Input: part model. Units: mm. Frame: model coordinates. A direction names the side the tool comes from. Coordinates: 2 decimals unless noted, no trailing zeros. Order: outer loops, then holes, each group sorted by start corner. A loop starts at its lowest first (then second) coordinate and runs counter-clockwise, first axis right, second up. Notation, with made-up numbers: (54, 18) - (85, 18) arc R13 ccw to (85, 30) - close; hole circle Ø3 at (4, 7). An arc over 180 degrees is marked (long way). One line per question, with ' | ' between items.
from build123d import *

# Parameters (mm, degrees)
SKETCH1_W            = 91
SKETCH1_H            = 71
BOSS_EXTRUDE1_DEPTH  = 3
SKETCH3_W            = 4
SKETCH3_H            = 4
CUT_EXTRUDE1_DEPTH   = 5
FILLET2_R            = 10
FILLET3_R            = 2
SKETCH4_W            = 15
SKETCH4_H            = 18
CUT_EXTRUDE2_DEPTH   = 5
SKETCH5_R            = 3.5
SKETCH5_R_2          = 2
BOSS_EXTRUDE2_DEPTH  = 7
LPATTERN1_COUNT      = 2
LPATTERN1_PITCH      = 81.28
LPATTERN1_COUNT_DIR2 = 2
LPATTERN1_PITCH_DIR2 = 60.96
FILLET4_R            = 2
BOSS_EXTRUDE4_DEPTH  = 9
FILLET5_R            = 1
BOSS_EXTRUDE5_DEPTH  = 5
FILLET6_R            = 1
SKETCH9_W            = 25
SKETCH9_H            = 3
BOSS_EXTRUDE6_DEPTH  = 7
FILLET7_R            = 1
SKETCH10_W           = 12
SKETCH10_H           = 14
CUT_EXTRUDE3_DEPTH   = 5
FILLET8_R            = 1
CUT_EXTRUDE4_REACH   = 60.57
SKETCH11_W           = 12
SKETCH11_H           = 5
FILLET9_R            = 1
SKETCH12_W           = 2
SKETCH12_H           = 31
BOSS_EXTRUDE7_DEPTH  = 5
FILLET10_R           = 0.5


# Some blends are built 0.0001 mm under size
with BuildPart() as part:
    # Sketch1 → Boss-Extrude1 (new body)
    with BuildSketch(Plane.XY):
        Rectangle(SKETCH1_W, SKETCH1_H)
    extrude(amount=BOSS_EXTRUDE1_DEPTH)

    # Sketch3 → Cut-Extrude1 (cut)
    with BuildSketch(Plane(origin=(0, 0, 0), x_dir=(-1, 0, 0), z_dir=(0, 0, -1))):
        with Locations((-43.5, 33.5)):
            Rectangle(SKETCH3_W, SKETCH3_H)
        with Locations((43.5, -33.5)):
            Rectangle(SKETCH3_W, SKETCH3_H)
    extrude(amount=-CUT_EXTRUDE1_DEPTH, mode=Mode.SUBTRACT)

    # Fillet2
    # the kernel refuses this fillet: 10 mm, written as the material it adds along each edge
    with BuildSketch(Plane(origin=(-41.5, -31.5, 0), x_dir=(0, -1, 0), z_dir=(0, 0, 1))) as fillet2_piece_1:
        with BuildLine():
            CenterArc((8.782329983, -8.782329983), FILLET2_R, 118.570059811, 32.859880379)
            Line((0, -4), (0, 0))
            Line((0, 0), (4, 0))
        make_face()
    extrude(amount=3)
    with BuildSketch(Plane(origin=(41.5, 31.5, 0), x_dir=(1, 0, 0), z_dir=(0, 0, 1))) as fillet2_piece_2:
        with BuildLine():
            CenterArc((8.782329983, 8.782329983), FILLET2_R, 208.570059811, 32.859880379)
            Line((0, 4), (0, 0))
            Line((0, 0), (4, 0))
        make_face()
    extrude(amount=3)

    # Fillet3
    fillet3_edges = [part.edges().sort_by_distance(p)[0] for p in [
        (-45.5, 35.5, 1.5),
        (45.5, -35.5, 1.5),
    ]]
    fillet(fillet3_edges, radius=FILLET3_R)

    # Sketch4 → Cut-Extrude2 (cut)
    with BuildSketch(Plane.XY.offset(3)):
        with Locations((33, 16.5)):
            Rectangle(SKETCH4_W, SKETCH4_H)
    extrude(amount=-CUT_EXTRUDE2_DEPTH, mode=Mode.SUBTRACT)

    # Sketch5 → Boss-Extrude2 (add)
    with BuildSketch(Plane.XY.offset(3)):
        with Locations((-40, 30)):
            Circle(SKETCH5_R)
        with Locations((-40, 30)):
            Circle(SKETCH5_R_2, mode=Mode.SUBTRACT)
    boss_extrude2 = extrude(amount=BOSS_EXTRUDE2_DEPTH)

    # LPattern1: Boss-Extrude2 2 × 2
    with Locations(*[(i * LPATTERN1_PITCH, -j * LPATTERN1_PITCH_DIR2, 0) for i in range(LPATTERN1_COUNT) for j in range(LPATTERN1_COUNT_DIR2) if (i, j) != (0, 0)]):
        add(boss_extrude2)

    # Fillet4
    fillet4_edges = [part.edges().sort_by_distance(p)[0] for p in [
        (25.5, 7.5, 1.5),
        (25.5, 25.5, 1.5),
        (40.5, 25.5, 1.5),
        (40.5, 7.5, 1.5),
    ]]
    fillet(fillet4_edges, radius=FILLET4_R)

    # Sketch7 → Boss-Extrude4 (add)
    with BuildSketch(Plane(origin=(0, 0, 0), x_dir=(-1, 0, 0), z_dir=(0, 0, -1))):
        Polygon((-24.5, 2.1), (-18.5, 2.1), (-18.5, 5.1), (-27.5, 5.1), (-27.5, -20.5), (-24.5, -20.5), align=None)
    boss_extrude4 = extrude(amount=BOSS_EXTRUDE4_DEPTH)

    # Mirror1: Boss-Extrude4 across plane
    add(boss_extrude4.mirror(Plane(origin=(-0.5, 0, 0), x_dir=(0, 0, 1), z_dir=(1, 0, 0))))

    # Fillet5
    fillet5_edges = [part.edges().sort_by_distance(p)[0] for p in [
        (24.5, -20.5, -4.5),
        (24.5, 2.1, -4.5),
        (18.5, 2.1, -4.5),
        (18.5, 5.1, -4.5),
        (27.5, 5.1, -4.5),
        (27.5, -20.5, -4.5),
        (-25.5, 2.1, -4.5),
        (-25.5, -20.5, -4.5),
        (-28.5, -20.5, -4.5),
        (-28.5, 5.1, -4.5),
        (-19.5, 5.1, -4.5),
        (-19.5, 2.1, -4.5),
    ]]
    fillet(fillet5_edges, radius=FILLET5_R)

    # Sketch8 → Boss-Extrude5 (add)
    with BuildSketch(Plane(origin=(0, 0, 0), x_dir=(-1, 0, 0), z_dir=(0, 0, -1))):
        Polygon((-40.5, -11.5), (-40.5, -21.5), (-36.5, -21.5), (-36.5, -23.5), (-42.5, -23.5), (-42.5, -11.5), align=None)
    extrude(amount=BOSS_EXTRUDE5_DEPTH)

    # Fillet6
    fillet6_edges = [part.edges().sort_by_distance(p)[0] for p in [
        (40.5, -11.5, -2.5),
        (40.5, -21.5, -2.5),
        (42.5, -11.5, -2.5),
        (42.5, -23.5, -2.5),
        (36.5, -23.5, -2.5),
        (36.5, -21.5, -2.5),
    ]]
    fillet(fillet6_edges, radius=FILLET6_R - 0.0001)  # a hair under: the kernel refuses the full size

    # Sketch9 → Boss-Extrude6 (add)
    with BuildSketch(Plane(origin=(0, 0, 0), x_dir=(-1, 0, 0), z_dir=(0, 0, -1))):
        with Locations((13, 13.8)):
            Rectangle(SKETCH9_W, SKETCH9_H)
    extrude(amount=BOSS_EXTRUDE6_DEPTH)

    # Fillet7
    fillet7_edges = [part.edges().sort_by_distance(p)[0] for p in [
        (-0.5, 15.3, -3.5),
        (-0.5, 12.3, -3.5),
        (-25.5, 12.3, -3.5),
        (-25.5, 15.3, -3.5),
    ]]
    fillet(fillet7_edges, radius=FILLET7_R)

    # Sketch10 → Cut-Extrude3 (cut)
    with BuildSketch(Plane(origin=(0, 0, 0), x_dir=(-1, 0, 0), z_dir=(0, 0, -1))):
        with Locations((36.5, 16.5)):
            Rectangle(SKETCH10_W, SKETCH10_H)
    extrude(amount=-CUT_EXTRUDE3_DEPTH, mode=Mode.SUBTRACT)

    # Fillet8
    fillet8_edges = [part.edges().sort_by_distance(p)[0] for p in [
        (-30.5, 9.5, 1.5),
        (-30.5, 23.5, 1.5),
        (-42.5, 23.5, 1.5),
        (-42.5, 9.5, 1.5),
    ]]
    fillet(fillet8_edges, radius=FILLET8_R)

    # Sketch11 → Cut-Extrude4 (cut, up to next)
    with BuildSketch(Plane(origin=(0, 0, 0), x_dir=(-1, 0, 0), z_dir=(0, 0, -1)), mode=Mode.PRIVATE) as cut_extrude4_sk1:
        with Locations((36.5, -23)):
            Rectangle(SKETCH11_W, SKETCH11_H)
    cut_extrude4_tool1 = extrude(cut_extrude4_sk1.sketch, amount=-CUT_EXTRUDE4_REACH, mode=Mode.PRIVATE) & part.part
    add(cut_extrude4_tool1.solids().sort_by_distance((-36.5, -23, 0))[0], mode=Mode.SUBTRACT)

    # Fillet9
    fillet9_edges = [part.edges().sort_by_distance(p)[0] for p in [
        (-30.5, -25.5, 1.5),
        (-30.5, -20.5, 1.5),
        (-42.5, -20.5, 1.5),
        (-42.5, -25.5, 1.5),
    ]]
    fillet(fillet9_edges, radius=FILLET9_R)

    # Sketch12 → Boss-Extrude7 (add)
    with BuildSketch(Plane(origin=(0, 0, 0), x_dir=(-1, 0, 0), z_dir=(0, 0, -1))):
        with Locations((44.5, -10)):
            Rectangle(SKETCH12_W, SKETCH12_H)
    extrude(amount=BOSS_EXTRUDE7_DEPTH)

    # Fillet10
    fillet10_edges = [part.edges().sort_by_distance(p)[0] for p in [
        (-43.5, 5.5, -2.5),
        (-43.5, -25.5, -2.5),
        (-45.5, -25.5, -2.5),
        (-45.5, 5.5, -2.5),
    ]]
    fillet(fillet10_edges, radius=FILLET10_R)


solid = part.part
Item 1: Section A-A on x = -40. Return the cut outline in (y, z).
Data:
outline: (-35.5, 0) - (-25.5, 0) - (-25.5, 3) - (-27.46, 3) - (-27.46, 10) - (-28.96, 10) - (-28.96, 3) - (-32.96, 3) - (-32.96, 10) - (-34.46, 10) - (-34.46, 3) - (-35.5, 3) - close; (-20.5, 0) - (9.5, 0) - (9.5, 3) - (-20.5, 3) - close; (23.5, 0) - (35.5, 0) - (35.5, 3) - (33.5, 3) - (33.5, 10) - (32, 10) - (32, 3) - (28, 3) - (28, 10) - (26.5, 10) - (26.5, 3) - (23.5, 3) - close
Item 2: Section C-C on y = 20.5. Return the cut outline in (x, z).
Data:
outline: (-45.5, 0) - (-42.5, 0) - (-42.5, 3) - (-45.5, 3) - close; (-30.5, 0) - (25.5, 0) - (25.5, 3) - (-30.5, 3) - close; (40.5, 0) - (45.5, 0) - (45.5, 3) - (40.5, 3) - close
Item 3: Draft query along Y for faces 1 (the face through (39, -21.5, -2)), 2 (the face through (40.82, -27.49, 6.45)), 3 (the face through (-44, -10, -5)). Return one class per face: released by +Y, released by -Y, zero draft, split by the parting line, or undercut.
Data:
face 1: released by +Y | face 2: undercut | face 3: zero draft
Item 4: Section D-D on x = -17.5. Return the cut outline in (y, z).
Data:
outline: (-35.5, 0) - (12.3, 0) - (12.3, -7) - (15.3, -7) - (15.3, 0) - (35.5, 0) - (35.5, 3) - (-35.5, 3) - close
Item 5: Access query for faces 4 (the face through (40.5, -16, -2)), 5 (the face through (42.355, -29.274, 6.451)), 6 (the face through (39.93, 8.1, 1.48)). Directions: +Z, -Z, +X, -X, +Y, -Y. A direction counts if a zero-diameter tool reaches every point of the face in a straight line with its end or side. Return the directions, or none.
Data:
face 4: -Z, +Y | face 5: +Z | face 6: +Z, -Z
Item 6: Contact query for flat-ended pins moving along their axis: P1, Ø3.5, axis at x = -40, y = 30, coming from the +Z side; P2, Ø4.5, axis at y = -12.5, z = -3.5, coming from the +X side; P3, Ø0.8, axis at y = 3.5, z = -3, coming from the +X side. Output: stop coordinate, or through.
Data:
P1: z = 3 | P2: x = 42.5 | P3: x = 27.5
Item 7: Section B-B on z = 1.75. Count the separate pieces of the cut face and the enclosed holes in it, and give its area (3 significant figures).
Data:
separate pieces: 1 | enclosed holes: 3 | area: 5,950 mm^2
Item 8: Ray query, line 1 (X direction, y = -16, z = -4.5); line 2 (X direction, y = 1, z = -3.5); line 3 (Y direction, x = 41.28, z = 5.5). Return the intervals inside material, ascending.
Data:
line 1: -45.5 to -43.5, -28.5 to -25.5, 24.5 to 27.5, 40.5 to 42.5 | line 2: -45.5 to -43.5, -28.5 to -25.5, 24.5 to 27.5 | line 3: -34.46 to -32.96, -28.96 to -27.46, 26.5 to 28, 32 to 33.5
